Here's how the part is built. I have some questions about the finished solid (model axes, mm). Face numbers are marked on the shaded views. A direction names the side the tool comes from. Give positions to 0.01 mm unless a question says otherwise; leave off trailing zeros. Order: outer loops, then holes, each group sorted by start corner. A loop starts at its lowest first (then second) coordinate and runs counter-clockwise, first axis right, second up.
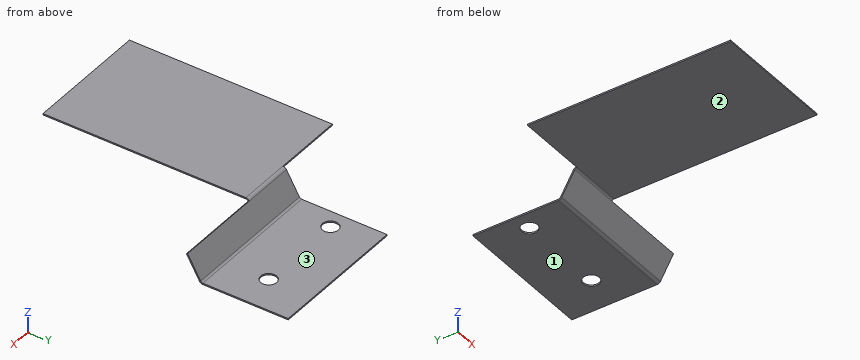
from build123d import *

# Parameters (mm, degrees)
SKETCH2_W               = 40
SKETCH2_H               = 25
SKETCH2_R               = 2.25
BASE_FLANGE1_DEPTH      = 0.4
EDGE_FLANGE1_DEPTH      = 40
EDGE_FLANGE1_2_DEPTH    = 40
EDGE_FLANGE2_DEPTH      = 15
EDGE_FLANGE2_START      = 0.4
EDGE_FLANGE2_PROFILE_W  = 35
EDGE_FLANGE2_PROFILE_H  = 57.343783684
EDGE_FLANGE2_FLAT_DEPTH = 0.4


# Read off the part's stored shape, not the designer's step: Edge-Flange1
# Sheet-metal steps are written as plain solids
with BuildPart() as part:
    # Sketch2 → Base-Flange1 (new body)
    with BuildSketch(Plane.XY):
        with Locations((20, 12.5)):
            Rectangle(SKETCH2_W, SKETCH2_H)
        with Locations((5, 12.5)):
            Circle(SKETCH2_R, mode=Mode.SUBTRACT)
        with Locations((30, 12.5)):
            Circle(SKETCH2_R, mode=Mode.SUBTRACT)
    extrude(amount=-BASE_FLANGE1_DEPTH)

    # Edge-Flange1 outline → Edge-Flange1 (cut)
    with BuildSketch(Plane.YZ):
        with BuildLine():
            ThreePointArc((0.887156424, -0.4), (0.410375552, -0.295165264), (0.021546812, 0))
            Line((0.021546812, 0), (0, 0))
            Line((0, 0), (0, -0.4))
            Line((0, -0.4), (0.887156424, -0.4))
        make_face()
    extrude(amount=EDGE_FLANGE1_DEPTH, mode=Mode.SUBTRACT)

    # Edge-Flange1 2 outline → Edge-Flange1 2 (add)
    with BuildSketch(Plane.YZ):
        with BuildLine():
            Line((-3.769059892, 6.52820323), (-0.09716805, 0.1683))
            ThreePointArc((-0.09716805, 0.1683), (-0.041630555, 0.081455507), (0.021546812, 0))
            Line((0.021546812, 0), (0.887156424, 0))
            ThreePointArc((0.887156424, 0), (0.518856424, 0.098685688), (0.249242111, 0.3683))
            Line((0.249242111, 0.3683), (-3.422649731, 6.72820323))
            Line((-3.422649731, 6.72820323), (-3.769059892, 6.52820323))
        make_face()
    extrude(amount=EDGE_FLANGE1_2_DEPTH)

    # Edge-Flange2 bend section (across the edge) → Edge-Flange2 (add)
    with BuildSketch(Plane(origin=(15, -3.981697996, 6.89650323), x_dir=(0, 0, -1), z_dir=(-1, 0, 0))):
        with BuildLine():
            Line((-0.4, 0.425276208), (0, 0.425276208))
            ThreePointArc((0, 0.425276208), (0.098685688, 0.056976208), (0.3683, -0.212638104))
            Line((0.3683, -0.212638104), (0.1683, -0.559048266))
            ThreePointArc((0.1683, -0.559048266), (-0.247724474, -0.143023792), (-0.4, 0.425276208))
        make_face()
    extrude(amount=EDGE_FLANGE2_DEPTH)

    # Edge-Flange2 profile (on flange) → Edge-Flange2 flat (add)
    with BuildSketch(Plane(origin=(0, -3.981697996, 6.89650323), x_dir=(-1, 0, 0), z_dir=(0, 0, 1)).offset(EDGE_FLANGE2_START)):
        with Locations((2.5, 29.09716805)):
            Rectangle(EDGE_FLANGE2_PROFILE_W, EDGE_FLANGE2_PROFILE_H)
    extrude(amount=-EDGE_FLANGE2_FLAT_DEPTH)


solid = part.part
Q1. I need wall thicknesses on L1, parallel to Y at x = 30, z = -0.2; L2, parallel to Z at x = -9.5, y = -15; L3, parallel to Z at x = 23.5, y = 19. Which ranges of each line are inside material? Lowest first, please.
Filled sheet:
L1: y = 0.24 to 10.25, 14.75 to 25
L2: z = 6.9 to 7.3
L3: z = -0.4 to 0
Q2. If we section it at D-D on z = 4.25: List the corners of the cut face in (x, y) for me, plus the area to 3 significant figures.
Filled sheet:
outline: (0, -2.45) - (40, -2.45) - (40, -1.99) - (0, -1.99) - close
area: 18.5 mm2
Q3. If we section it at A-A on x = 30: List the corners of the cut face in (y, z) for me.
Filled sheet:
outline: (-3.77, 6.53) - (-0.1, 0.17) arc R1.14 ccw to (0.89, -0.4) - (10.25, -0.4) - (10.25, 0) - (0.89, 0) arc R0.74 cw to (0.25, 0.37) - (-3.42, 6.73) - close; (14.75, -0.4) - (25, -0.4) - (25, 0) - (14.75, 0) - close
Q4. For the marked faces 1, 2 and 3, which set-ups out of +Z, -Z, +X, -X, +Y, -Y let a thin tool reach every point of the face, with its end or its side?
Filled sheet:
face 1: -Z, +X, -X, +Y, -Y
face 2: -Z, +X, -X, -Y
face 3: +Z, +X, -X, +Y
Q5. If we section it at B-B on y = 12.5: List the corners of the cut face in (x, z) for me, plus the area to 3 significant figures.
Filled sheet:
outline: (0, -0.4) - (2.75, -0.4) - (2.75, 0) - (0, 0) - close; (7.25, -0.4) - (27.75, -0.4) - (27.75, 0) - (7.25, 0) - close; (32.25, -0.4) - (40, -0.4) - (40, 0) - (32.25, 0) - close
area: 12.4 mm2
Q6. If we section it at C-C on x = 5: List the corners of the cut face in (y, z) for me.
Filled sheet:
outline: (-61.75, 6.9) - (-4.41, 6.9) arc R0.74 cw to (-3.77, 6.53) - (-0.1, 0.17) arc R1.14 ccw to (0.89, -0.4) - (10.25, -0.4) - (10.25, 0) - (0.89, 0) arc R0.74 cw to (0.25, 0.37) - (-3.42, 6.73) arc R1.14 ccw to (-4.41, 7.3) - (-61.75, 7.3) - close; (14.75, -0.4) - (25, -0.4) - (25, 0) - (14.75, 0) - close
Q7. I'm going to push flat-ended pins straight in: P1, Ø1.5, axis at x = -10, y = -31.5, coming from the -Z side; P2, Ø4, axis at y = 8, z = 2.5, coming from the -X side; P3, Ø5, axis at x = 30, y = 12.5, coming from the +Z side; P4, Ø4, axis at x = 16.5, y = -44, coming from the +Z side. Where does each tip first touch, or does it pass through?
Filled sheet:
P1: stops at z = 6.9
P2: passes through
P3: stops at z = 0
P4: stops at z = 7.3
